The model under review builds one solid part; all positions refer to its coordinate system, in mm. Round coordinates to 2 decimals unless told otherwise and drop trailing zeros. Order: outer loops, then holes, each group sorted by start corner. A loop starts at its lowest first (then second) coordinate and runs counter-clockwise, first axis right, second up. Notation, with made-up numbers: M -35.75,-18 L -10.75,-18 A22 ccw -10.75,-8 Z; hole C -16.75,-22.5 d9. An arc over 180 degrees is marked long. Answer as a JSON object with one key per item and string values. Group by question number.
1) Consider section C-C, the plane x = -58. Write out the cut boundary in (y, z) (3 decimals).
2) To check wall thickness, follow line 1 (X direction, y = 1.75, z = 4.5) (3 decimals); line 2 (Z direction, x = -1.5, y = 2.25); line 3 (X direction, y = 2.3, z = 70). State the ranges of each line that lie inside material, in increasing order.
3) Insertion check: pin 1 Ø11.5 at (x, z) = (47.23, 105.33) entering from +Y; pin 2 Ø1.5 at (y, z) = (3, -39.5) entering from -X. Each pin has a flat end and moves straight along its axis. Give the tip position at first contact, or say it passes through.
4) Consider section B-B, the plane z = 44. Write out the cut boundary in (x, y) (3 decimals).
5) Consider section A-A, the plane x = -97. Write out the cut boundary in (y, z) (3 decimals), then the cut area to 3 significant figures.
6) The part is to be moulded in two halves that separate along Z. For faces 1 (the flat face through (-29.4, 0, 78.3)), 2 (the cylindrical face through (80.301, 1.565, -83.833)), 3 (the cylindrical face through (53.011, 1.565, 66.957)), say which applies: +Z half, -Z half, draft (parallel to the pull), parting line (faces both ways), or undercut.
7) Consider section D-D, the plane y = 1.25. Count the separate pieces of the cut face and the enclosed holes in it, then the cut area to 3 significant figures.
```python
from build123d import *

# Parameters (mm, degrees)
SKETCH1_R           = 84.7725
SKETCH1_R_2         = 6.35
BOSS_EXTRUDE1_DEPTH = 3.175


with BuildPart() as part:
    # Sketch1 → Boss-Extrude1 (new body)
    with BuildSketch(Plane(origin=(0, 0, 0), x_dir=(1, 0, 0), z_dir=(0, 1, 0))):
        with BuildLine():
            Line((16.751670796, 110.565701996), (-3.568329204, 110.565701996))
            ThreePointArc((-3.568329204, 110.565701996), (-76.150812933, 83.28188355), (-112.788329204, 14.942172584))
            Line((-112.788329204, 14.942172584), (-112.788329204, -118.034298004))
            Line((-112.788329204, -118.034298004), (105.651670796, -118.034298004))
            Line((105.651670796, -118.034298004), (105.651670796, 21.665701996))
            ThreePointArc((105.651670796, 21.665701996), (79.613463644, 84.527494844), (16.751670796, 110.565701996))
        make_face()
        with Locations((-3.568329204, 2.615701996)):
            Circle(SKETCH1_R, mode=Mode.SUBTRACT)
        with Locations((-98.436496296, -9.450545062)):
            Circle(SKETCH1_R_2, mode=Mode.SUBTRACT)
        with Locations((-54.368329204, -105.334298004)):
            Circle(SKETCH1_R_2, mode=Mode.SUBTRACT)
        with Locations((47.231670796, -105.334298004)):
            Circle(SKETCH1_R_2, mode=Mode.SUBTRACT)
        with Locations((32.954821104, 90.521109481)):
            Circle(SKETCH1_R_2, mode=Mode.SUBTRACT)
        with Locations((53.837154897, -73.252936495)):
            Circle(SKETCH1_R_2, mode=Mode.SUBTRACT)
    extrude(amount=BOSS_EXTRUDE1_DEPTH)


solid = part.part
```
Results list:
{
 "1": {"outline": "M 0,-96.182 L 3.175,-96.182 L 3.175,-67.605 L 0,-67.605 Z; M 0,62.373 L 3.175,62.373 L 3.175,100.125 L 0,100.125 Z; M 0,110.543 L 3.175,110.543 L 3.175,118.034 L 0,118.034 Z"},
 "2": {"line 1": "-112.788 to -102.413, -94.46 to -88.042, 80.905 to 105.652", "line 2": "-110.57 to -87.36, 82.13 to 118.03", "line 3": "-112.79 to -47.31, 40.17 to 48.38, 59.29 to 105.65"},
 "3": {"pin 1": "through", "pin 2": "x = -106.86"},
 "4": {"outline": "M -112.788,0 L -74.373,0 L -74.373,3.175 L -112.788,3.175 Z; M 67.237,0 L 105.652,0 L 105.652,3.175 L 67.237,3.175 Z"},
 "5": {"outline": "M 0,-58.788 L 3.175,-58.788 L 3.175,3.265 L 0,3.265 Z; M 0,15.636 L 3.175,15.636 L 3.175,118.034 L 0,118.034 Z", "area": "522 mm^2"},
 "6": {"face 1": "draft", "face 2": "-Z half", "face 3": "undercut"},
 "7": {"separate pieces": "1", "enclosed holes": "6", "area": "22,500 mm^2"}
}
